Check sheet for the drawn part. Datum: minimum x, y, z corner. Units: mm. A direction names the side the tool comes from. Give positions to 0.01 mm unless a question says otherwise; leave off trailing zeros. Order: outer loops, then holes, each group sorted by start corner. A loop starts at its lowest first (then second) coordinate and runs counter-clockwise, first axis right, second up. Notation, with made-up numbers: (-29, -34.75) -> (23, -34.75) arc R9 cw to (23, -20.75) -> close; hole circle Ø2 at (-0.5, 25). An arc over 180 degrees is marked (long way). One line per question, with ' | ' between items. Start each with the question number.
Q1. Section check C-C on y = 38. Record the cut outline in (x, z).
Q2. Section check A-A on z = 21. Record the cut outline in (x, y).
Q3. Section check D-D on y = 29.5. Record the cut outline in (x, z).
Q4. Go/stop test with flat-tipped pins: pin 1 (2 mm diameter, centred on x = 49, y = 33.5, fed in from -Z); pin 2 (14 mm diameter, centred on y = 38, z = 21, fed in from -X); pin 3 (22 mm diameter, centred on y = 41, z = 24.5, fed in from +X). Record where each tip stops, or that it passes through.
Q5. Mould release check, pull along X, two halves, no side actions. Record for the marked faces 6, 7 and 8: released by +X, released by -X, zero draft, split by the parting line, or undercut.
Q6. Access from +Z, -Z, +X, -X, +Y, -Y to the whole of each face (thin tool, end or side, straight path). Record for the marked faces 1, 2, 3, 4 and 5.
Q7. Section check B-B on x = 54. Record the cut outline in (y, z).
Q8. Material ranges on probe 1 along Y at (x, z) = (41, 21); probe 2 along Y at (x, z) = (60, 36.5); probe 3 along X at (y, z) = (29, 21), recorded low to high. Write a range as [from, to].
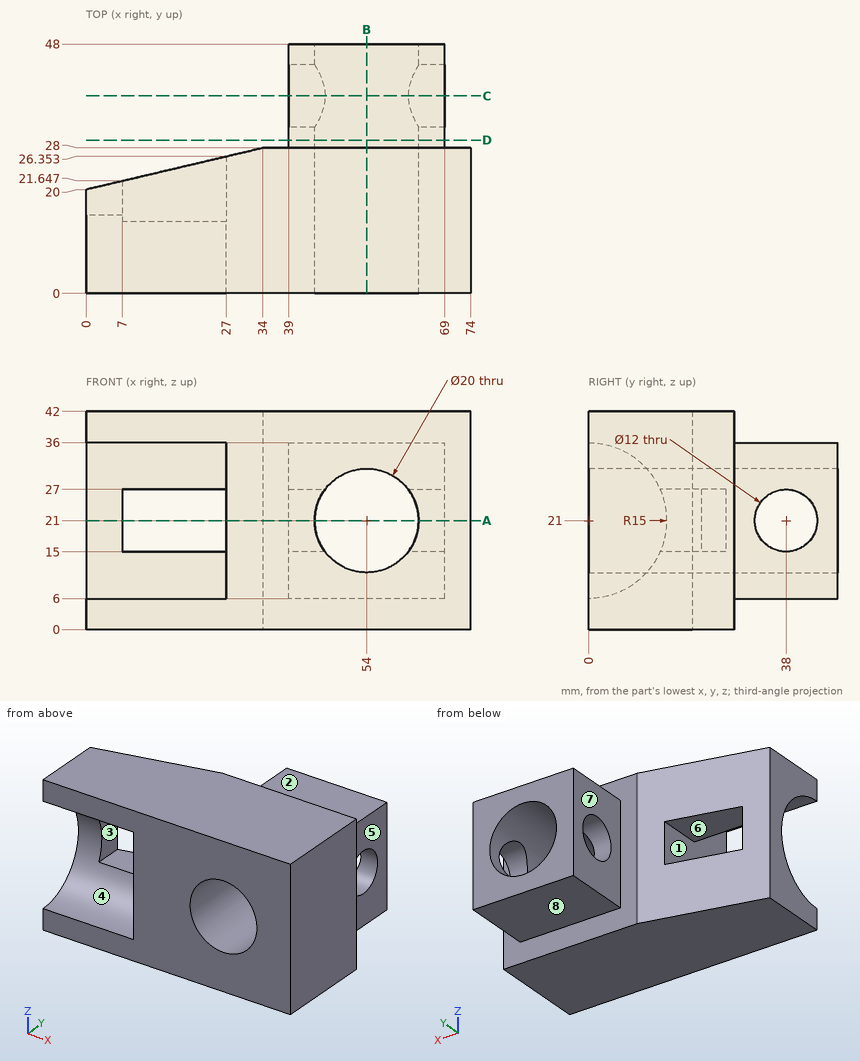
Filled in:
1) outline: (39, 6) -> (69, 6) -> (69, 15) -> (62, 15) arc R10 cw to (46, 15) -> (39, 15) -> close; (39, 27) -> (46, 27) arc R10 cw to (62, 27) -> (69, 27) -> (69, 36) -> (39, 36) -> close
2) outline: (0, 15) -> (7, 15) -> (7, 21.65) -> (0, 20) -> close; (27, 0) -> (44, 0) -> (44, 32) -> (39, 32) -> (39, 28) -> (34, 28) -> (27, 26.35) -> close; (39, 44) -> (44, 44) -> (44, 48) -> (39, 48) -> close; (64, 0) -> (74, 0) -> (74, 28) -> (69, 28) -> (69, 32) -> (64, 32) -> close; (64, 44) -> (69, 44) -> (69, 48) -> (64, 48) -> close
3) outline: (39, 6) -> (69, 6) -> (69, 36) -> (39, 36) -> close; hole circle Ø20 at (54, 21)
4) pin 1: z = 6 | pin 2: x = 39 | pin 3: x = 69
5) face 6: undercut | face 7: released by -X | face 8: zero draft
6) face 1: -Y | face 2: +Z, +X, -X, +Y | face 3: +Y, -Y | face 4: -X, -Y | face 5: +Z, -Z, +X, +Y
7) outline: (0, 0) -> (28, 0) -> (28, 6) -> (48, 6) -> (48, 11) -> (0, 11) -> close; (0, 31) -> (48, 31) -> (48, 36) -> (28, 36) -> (28, 42) -> (0, 42) -> close
8) probe 1: [0, 32], [44, 48] | probe 2: [0, 28] | probe 3: [39, 44], [64, 69]
